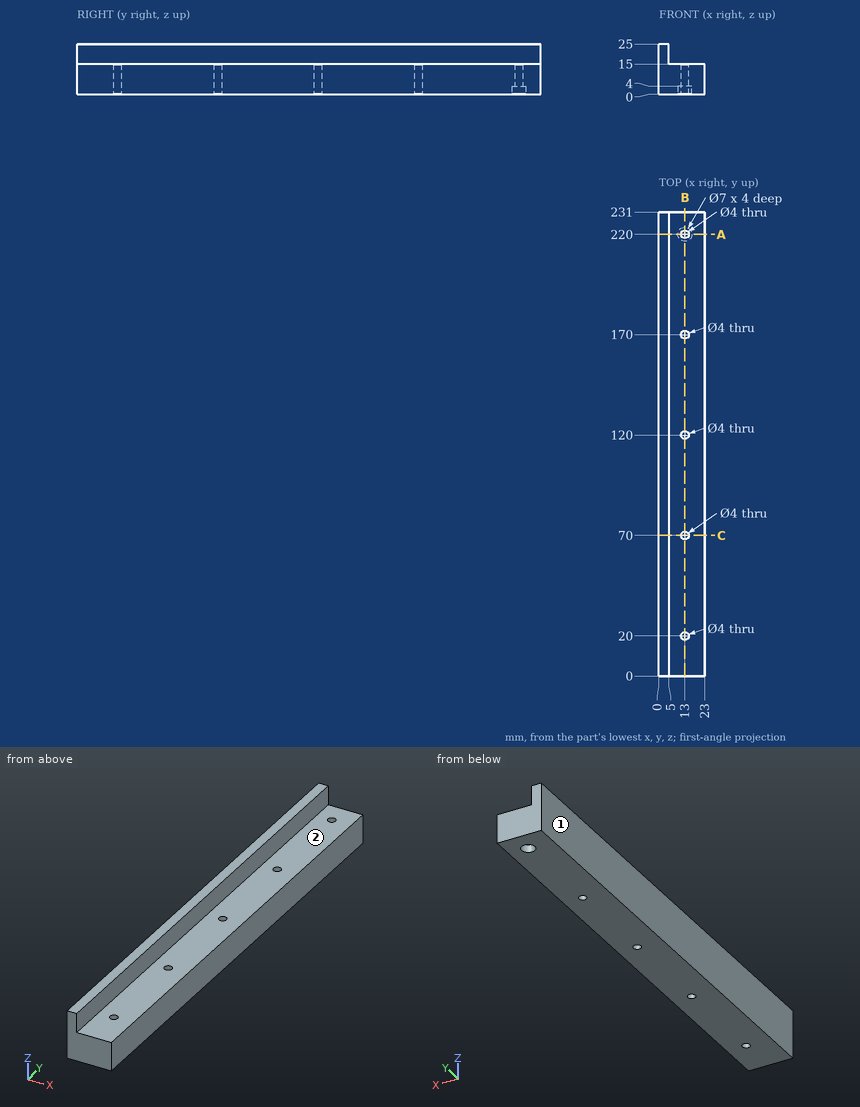
Can you work these out from the drawing? Everything is in mm from the part's minimum corner. A direction names the side the tool comes from. Give positions to 0.01 mm unless a question says otherwise; leave off trailing zeros. Order: outer loops, then holes, each group sorted by start corner. A loop starts at its lowest first (then second) coordinate and runs counter-clockwise, first axis right, second up. Notation, with made-up numbers: M 52.25,68 L 68.25,68 A38 cw 68.25,107 Z; hole C 62.25,65 d6. An arc over 180 degrees is marked long. Use a Markdown table: item, result. Add a question column.
Item 1: For the marked faces 1 and 2, which set-ups out of +Z, -Z, +X, -X, +Y, -Y let a thin tool reach every point of the face, with its end or its side?
Item 2: Suppose I cut it at C-C (y = 70). List the corners of the cut face in (x, z) for me.
Item 3: Suppose I cut it at A-A (y = 220). List the corners of the cut face in (x, z) for me, then the cut area to 3 significant figures.
Item 4: Will these pins go through, and if not, where does the flat tip stop? pin 1 (3 mm diameter, centred on x = 15, y = 197, fed in from +Z); pin 2 (5.5 mm diameter, centred on x = 13, y = 220, fed in from -Z); pin 3 (6 mm diameter, centred on y = 49.5, z = 20.5, fed in from +X).
Item 5: If I drill on L1, parallel to Y at x = 13, z = 1.2; L2, parallel to Y at x = 13, z = 5.75; L3, parallel to X at y = 120, z = 11.25, over which ranges is the centre line in solid material (lowest first)? Write a range as [from, to].
Item 6: Suppose I cut it at B-B (x = 13). List the corners of the cut face in (y, z) for me.
Answer sheet:
| question | item | result |
|---|---|---|
| 1 | face 1 | +Z, -Z, -X, +Y, -Y |
| 1 | face 2 | +Z, +X, +Y, -Y |
| 2 | outline | M 0,0 L 11,0 L 11,15 L 5,15 L 5,25 L 0,25 Z; M 15,0 L 23,0 L 23,15 L 15,15 Z |
| 3 | outline | M 0,0 L 9.5,0 L 9.5,4 L 11,4 L 11,15 L 5,15 L 5,25 L 0,25 Z; M 15,4 L 16.5,4 L 16.5,0 L 23,0 L 23,15 L 15,15 Z |
| 3 | area | 323 mm² |
| 4 | pin 1 | stops at z = 15 |
| 4 | pin 2 | stops at z = 4 |
| 4 | pin 3 | stops at x = 5 |
| 5 | L1 | y = [0, 18], [22, 68], [72, 118], [122, 168], [172, 216.5], [223.5, 231] |
| 5 | L2 | y = [0, 18], [22, 68], [72, 118], [122, 168], [172, 218], [222, 231] |
| 5 | L3 | x = [0, 11], [15, 23] |
| 6 | outline | M 0,0 L 18,0 L 18,15 L 0,15 Z; M 22,0 L 68,0 L 68,15 L 22,15 Z; M 72,0 L 118,0 L 118,15 L 72,15 Z; M 122,0 L 168,0 L 168,15 L 122,15 Z; M 172,0 L 216.5,0 L 216.5,4 L 218,4 L 218,15 L 172,15 Z; M 222,4 L 223.5,4 L 223.5,0 L 231,0 L 231,15 L 222,15 Z |
